```python
from build123d import *

# Parameters (mm, degrees)
F1_DEPTH  = 4
F2_DEPTH  = 2
F3_START  = 2
F3_DEPTH  = 2
F4_SIZE   = 1.99999
F6_START  = 3.75
F5_R      = 2
F6_DEPTH  = 0.25
F7_DEPTH  = 3.5
F8_DEPTH  = 3.5
F9_DEPTH  = 3
F10_DEPTH = 3.25
F11_DEPTH = 3


# Not quite as in the source:
# - a fillet or chamfer is up to 0.001 mm smaller than in the source, because OpenCascade refuses the exact size


with BuildPart() as f1:
    # F0 (on Top) → F1 (new body)
    with BuildSketch(Plane.XY):
        Polygon((32.7846783229, 14.824549064), (4.8026783229, 63.2907947614), (-23.1793216771, 14.824549064), align=None)
        Polygon((-19.715220062, 16.824549064), (4.8026783229, 59.2907947614), (29.3205767077, 16.824549064), align=None, mode=Mode.SUBTRACT)
    extrude(amount=F1_DEPTH)

    # F0 (on Top) → F2 (join)
    with BuildSketch(Plane.XY):
        Polygon((37.1148053418, 12.324549064), (4.8026783229, 68.2907947614), (-27.509448696, 12.324549064), align=None)
        Polygon((-23.1793216771, 14.824549064), (4.8026783229, 63.2907947614), (32.7846783229, 14.824549064), align=None, mode=Mode.SUBTRACT)
    extrude(amount=F2_DEPTH)

    # F0 (on Top) → F3 (join)
    with BuildSketch(Plane.XY.offset(F3_START)):
        Polygon((29.3205767077, 16.824549064), (4.8026783229, 59.2907947614), (-19.715220062, 16.824549064), align=None)
    extrude(amount=F3_DEPTH)

    # F4 (size 2 in the source; OpenCascade refuses exactly that, so slightly less here)
    f4_edges = [f1.edges().sort_by_distance(p)[0] for p in [
        (4.802678, 16.824549, 0),
        (-7.456271, 38.057672, 0),
        (17.061628, 38.057672, 0),
    ]]
    chamfer(f4_edges, length=F4_SIZE)

    # F5 (on face) → F6 (cut)
    with BuildSketch(Plane.XY.offset(F6_START)):
        with BuildLine():
            Line((15.8012454512, 40.2407176847), (14.8071694273, 41.9625078646))
            ThreePointArc((14.8071694273, 41.9625078646), (12.0675004242, 39.2368445398), (15.801257126, 40.2338840067))
            ThreePointArc((15.801257126, 40.2338840067), (15.8012542073, 40.2373008507), (15.8012454512, 40.2407176847))
        make_face()
        with BuildLine():
            Line((17.0693753854, 23.8813530259), (14.9441122519, 35.3662478082))
            ThreePointArc((14.9441122519, 35.3662478082), (14.2087911946, 35.2505200844), (13.4644377158, 35.2452416378))
            Line((13.4644377158, 35.2452416378), (12.8494622186, 26.1368211359))
            Line((12.8494622186, 26.1368211359), (15.8132929355, 24.552706629))
            Line((15.8132929355, 24.552706629), (17.0693753854, 23.8813530259))
        make_face()
        with BuildLine():
            ThreePointArc((9.6781818277, 43.0623553402), (10.154568974, 43.6546537332), (10.7152328484, 44.1678964823))
            Line((10.7152328484, 44.1678964823), (5.5434275419, 50.7608279586))
            Line((5.5434275419, 50.7608279586), (5.1609951292, 49.6271412781))
            Line((5.1609951292, 49.6271412781), (4.2115291581, 46.8125343323))
            Line((4.2115291581, 46.8125343323), (9.6781818277, 43.0623553402))
        make_face()
        with BuildLine():
            Line((-13.4587365793, 16.824549064), (-6.1025659626, 16.824549064))
            Line((-6.1025659626, 16.824549064), (-3.819498702, 19.0105444595))
            Line((-3.819498702, 19.0105444595), (-1.2189327972, 21.5005390346))
            Line((-1.2189327972, 21.5005390346), (-7.725601985, 22.742720621))
            ThreePointArc((-7.725601985, 22.742720621), (-9.2656609828, 20.6555454959), (-11.8573356204, 20.5492238495))
            Line((-11.8573356204, 20.5492238495), (-13.4587365793, 16.824549064))
        make_face()
        with BuildLine():
            Line((3.6860700174, 34.755180139), (9.4204377363, 37.8238173116))
            ThreePointArc((9.4204377363, 37.8238173116), (9.2694965624, 38.1212680469), (9.1387235678, 38.4281207834))
            Line((9.1387235678, 38.4281207834), (0.9941436583, 35.2838113904))
            Line((0.9941436583, 35.2838113904), (-2.8154677711, 33.8130667806))
            Line((-2.8154677711, 33.8130667806), (1.0452440474, 33.3419926465))
            Line((1.0452440474, 33.3419926465), (3.6860700174, 34.755180139))
        make_face()
        with Locations((-10.6723830104, 23.3052875847)):
            Circle(F5_R)
    extrude(amount=F6_DEPTH, mode=Mode.SUBTRACT)

    # F5 (on face) → F7 (cut)
    with BuildSketch(Plane.XY):
        with BuildLine():
            Line((15.8012454512, 40.2407176847), (14.8071694273, 41.9625078646))
            ThreePointArc((14.8071694273, 41.9625078646), (12.0675004242, 39.2368445398), (15.801257126, 40.2338840067))
            ThreePointArc((15.801257126, 40.2338840067), (15.8012542073, 40.2373008507), (15.8012454512, 40.2407176847))
        make_face()
        with Locations((-10.6723830104, 23.3052875847)):
            Circle(F5_R)
    extrude(amount=F7_DEPTH, mode=Mode.SUBTRACT)

    # F5 (on face) → F8 (cut)
    with BuildSketch(Plane.XY):
        with BuildLine():
            Line((3.6860700174, 34.755180139), (9.4204377363, 37.8238173116))
            ThreePointArc((9.4204377363, 37.8238173116), (9.2694965624, 38.1212680469), (9.1387235678, 38.4281207834))
            Line((9.1387235678, 38.4281207834), (0.9941436583, 35.2838113904))
            Line((0.9941436583, 35.2838113904), (-2.8154677711, 33.8130667806))
            Line((-2.8154677711, 33.8130667806), (1.0452440474, 33.3419926465))
            Line((1.0452440474, 33.3419926465), (3.6860700174, 34.755180139))
        make_face()
        with BuildLine():
            Line((17.0693753854, 23.8813530259), (14.9441122519, 35.3662478082))
            ThreePointArc((14.9441122519, 35.3662478082), (14.2087911946, 35.2505200844), (13.4644377158, 35.2452416378))
            Line((13.4644377158, 35.2452416378), (12.8494622186, 26.1368211359))
            Line((12.8494622186, 26.1368211359), (15.8132929355, 24.552706629))
            Line((15.8132929355, 24.552706629), (17.0693753854, 23.8813530259))
        make_face()
        with BuildLine():
            Line((-13.4587365793, 16.824549064), (-6.1025659626, 16.824549064))
            Line((-6.1025659626, 16.824549064), (-3.819498702, 19.0105444595))
            Line((-3.819498702, 19.0105444595), (-1.2189327972, 21.5005390346))
            Line((-1.2189327972, 21.5005390346), (-7.725601985, 22.742720621))
            ThreePointArc((-7.725601985, 22.742720621), (-9.2656609828, 20.6555454959), (-11.8573356204, 20.5492238495))
            Line((-11.8573356204, 20.5492238495), (-13.4587365793, 16.824549064))
        make_face()
        with BuildLine():
            ThreePointArc((9.6781818277, 43.0623553402), (10.154568974, 43.6546537332), (10.7152328484, 44.1678964823))
            Line((10.7152328484, 44.1678964823), (5.5434275419, 50.7608279586))
            Line((5.5434275419, 50.7608279586), (5.1609951292, 49.6271412781))
            Line((5.1609951292, 49.6271412781), (4.2115291581, 46.8125343323))
            Line((4.2115291581, 46.8125343323), (9.6781818277, 43.0623553402))
        make_face()
    extrude(amount=F8_DEPTH, mode=Mode.SUBTRACT)

    # F5 (on face) → F9 (cut)
    with BuildSketch(Plane.XY):
        with BuildLine():
            Line((19.8564007878, 24.4885329157), (15.5959561349, 35.5670804467))
            ThreePointArc((15.5959561349, 35.5670804467), (15.2734627879, 35.4555359146), (14.9441122519, 35.3662478082))
            Line((14.9441122519, 35.3662478082), (17.0693753854, 23.8813530259))
            Line((17.0693753854, 23.8813530259), (15.8132929355, 24.552706629))
            Line((15.8132929355, 24.552706629), (17.4690298736, 20.0315453112))
            Line((17.4690298736, 20.0315453112), (19.8564007878, 24.4885329157))
        make_face()
        Polygon((-6.1025659626, 16.824549064), (1.2875116271, 16.824549064), (1.7734020948, 17.1169545501), (-3.819498702, 19.0105444595), align=None)
        with BuildLine():
            Line((5.785849411, 33.66388008), (9.9342960343, 37.064244924))
            ThreePointArc((9.9342960343, 37.064244924), (9.6599157648, 37.4322252607), (9.4204377363, 37.8238173116))
            Line((9.4204377363, 37.8238173116), (3.6860700174, 34.755180139))
            Line((3.6860700174, 34.755180139), (5.785849411, 33.66388008))
        make_face()
        with BuildLine():
            ThreePointArc((11.5326481984, 44.6896009562), (11.8941525727, 44.8558913869), (12.2677356256, 44.9929082563))
            Line((12.2677356256, 44.9929082563), (11.2701070238, 48.0888796571))
            Line((11.2701070238, 48.0888796571), (7.7075759005, 54.2593645662))
            Line((7.7075759005, 54.2593645662), (6.1958078295, 55.1715530455))
            Line((6.1958078295, 55.1715530455), (7.7216781624, 52.1746300315))
            Line((7.7216781624, 52.1746300315), (11.5326481984, 44.6896009562))
        make_face()
        with BuildLine():
            ThreePointArc((-12.7082549566, 21.1018299793), (-12.079105038, 25.9550296735), (-7.7066088949, 23.7571547066))
            Line((-7.7066088949, 23.7571547066), (-6.6805827438, 23.5612770993))
            ThreePointArc((-6.6805827438, 23.5612770993), (-12.5480123805, 26.8382770364), (-13.1208381636, 20.1422088056))
            Line((-13.1208381636, 20.1422088056), (-12.7082549566, 21.1018299793))
        make_face()
    extrude(amount=F9_DEPTH, mode=Mode.SUBTRACT)

    # F10 (cut): faces of the model
    f10_faces = [f1.faces().sort_by_distance(p)[0] for p in [
        (9.5592668565, 49.7626778986, 3),
        (6.8730240158, 35.6258562625, 3),
        (-2.519612135, 17.5665266523, 3),
        (17.3422888297, 27.0693911728, 3),
    ]]
    extrude(f10_faces, amount=-F10_DEPTH, mode=Mode.SUBTRACT)

    # F5 (on face) → F11 (cut)
    with BuildSketch(Plane.XY):
        with BuildLine():
            ThreePointArc((9.1387235678, 38.4281207834), (8.9697402045, 38.9468547775), (8.8582790135, 39.4809116441))
            Line((8.8582790135, 39.4809116441), (1.4540485572, 38.196541369))
            Line((1.4540485572, 38.196541369), (0.9941436583, 35.2838113904))
            Line((0.9941436583, 35.2838113904), (9.1387235678, 38.4281207834))
        make_face()
        with BuildLine():
            ThreePointArc((10.7152328484, 44.1678964823), (11.1112630591, 44.4486119837), (11.5326481984, 44.6896009562))
            Line((11.5326481984, 44.6896009562), (7.7216781624, 52.1746300315))
            Line((7.7216781624, 52.1746300315), (3.6355266348, 51.2855537236))
            Line((3.6355266348, 51.2855537236), (5.1609951292, 49.6271412781))
            Line((5.1609951292, 49.6271412781), (5.5434275419, 50.7608279586))
            Line((5.5434275419, 50.7608279586), (10.7152328484, 44.1678964823))
        make_face()
    extrude(amount=F11_DEPTH, mode=Mode.SUBTRACT)


solid = f1.part
```
The model under review builds one solid part; all positions refer to its coordinate system, in mm. A direction names the side the tool comes from. Round coordinates to 2 decimals unless told otherwise and drop trailing zeros. Loops run counter-clockwise (first coordinate to the right, second up) from the corner with the lowest first, then second, coordinate; pieces in that order, holes last. Notation, with made-up numbers: (17, -17.75) - (53, -17.75) arc R19 cw to (53, -13.75) - close; hole circle Ø6 at (68, -28). An arc over 180 degrees is marked (long way). Write each question's results on one line, items separated by ' | '. Start each with the question number.
Q1. Tool access review of faces 1 (the flat face through (17.756, 29.95, 2.986)), 2 (the flat face through (-11, 23, 3.75)), 3 (the flat face through (14, 40, 3.5)): name each direction out of +Z, -Z, +X, -X, +Y, -Y from which nothing blocks a thin tool from reaching the whole face with its end or side.
Q2. Draft analysis for pull direction Y (two halves, no side actions). For faces 4 (the flat face through (-0.98, 18.05, 2.99)), 5 (the flat face through (-8.99, 39.4, 2.99)), 6 (the flat face through (4, 34, 4)), state which applies: pulls with the +Y half, pulls with the -Y half, needs draft (parallel to the pull), parting line crosses it, or undercut.
Q3. Take a section at C-C on z = 0.9. Give the boundary of the cut face in (x, y).
Q4. Wall thickness on line 1 along Y through (x, z) = (7.5, 3.35); line 2 along Y through (x, z) = (-3, 2.6); line 3 along X through (y, z) = (16.5, 1.5): over which ranges is each line inside the solid? List them lowest first. Write a range as [from, to].
Q5. Insertion check: P1, Ø1.5, axis at x = 6.5, y = 36, coming from the -Z side; P2, Ø1, axis at x = 7, z = 3.5, coming from the +Y side; P3, Ø1.5, axis at y = 23, z = 1, coming from the -X side. Each pin has a flat end and moves straight along its axis. Give the tip position at first contact, or say it passes through.
Data:
1) face 1: +Z, -Z | face 2: +Z | face 3: -Z
2) face 4: undercut | face 5: pulls with the +Y half | face 6: needs draft
3) outline: (-27.51, 12.32) - (37.11, 12.32) - (4.8, 68.29) - close; hole (-21.62, 15.72) - (31.23, 15.72) - (4.8, 61.49) - close
4) line 1: y = [14.82, 35.07], [37.8, 44.56], [48.27, 52.61], [54.38, 58.62] | line 2: y = [14.82, 16.82], [18.73, 19.8], [21.84, 49.78] | line 3: x = [-25.1, -20.48], [30.09, 34.7]
5) P1: stops at z = 3.5 | P2: stops at y = 60.35 | P3: stops at x = -21.78
